Geometry: final body of the model. Coordinates: model frame, mm. A direction names the side the tool comes from. Round coordinates to 2 decimals unless told otherwise and drop trailing zeros. Write each loop counter-clockwise with the first axis right and the second up, starting at its lowest first coordinate (ties: lowest second). Pieces come first, ordered by that corner, then holes. Notation, with made-up numbers: (78.5, 38) -> (89.5, 38) arc R13 ccw to (89.5, 44) -> close; hole circle Ø7 at (2, 17.5). An arc over 180 degrees is marked (long way). Use one line per item in the form item = value. Start each with the question number.
1. Cut plane C-C, the plane x = 11. Return the cut outline in (y, z).
2. Line query: L1, parallel to Y at x = 16.5, z = 3.5; L2, parallel to X at y = 63, z = 5; L3, parallel to Y at x = -1.5, z = 4.5. Output: solid intervals per line, ascending.
3. Cut plane B-B, the plane x = 0. Return the cut outline in (y, z), plus the area to 3 significant figures.
4. Reachability of faces 1 (the face through (12.22, 64.21, -17.55)), 2 (the face through (21.209, 68, 0)), 3 (the face through (20.871, 63.634, 20.891)) from +Z, -Z, +X, -X, +Y, -Y: full face, straight path, thin tool, end or side. Return the list, or none.
5. Cut plane D-D, the plane z = 8. Return the cut outline in (x, y), plus the area to 3 significant figures.
6. Draft query along Z for faces 4 (the face through (8.598, 64, 0)), 5 (the face through (-21.209, 68, 0)), 6 (the face through (0.3, 63.6, -21.2)), 7 (the face through (0, 0, 0)). Return one class per face: pulls with the +Z half, pulls with the -Z half, needs draft (parallel to the pull), parting line crosses it, or undercut.
7. Pin query (flat end, axial travel): pin 1 Ø4 at (x, z) = (8.5, -3.5) entering from -Y; pin 2 Ø5 at (x, y) = (-2, 61.5) entering from -Z; pin 3 Ø2 at (x, z) = (-17.5, 14.5) entering from +Y. Return the tip coordinate at first contact, or that it passes through.
8. Cut plane A-A, the plane z = 0. State how many separate pieces and enclosed holes the cut face has, plus the area to 3 significant figures.
```python
from build123d import *

# Parameters (mm, degrees)
SKETCH1_R           = 1.9939
BOSS_EXTRUDE1_DEPTH = 62.8904
SKETCH2_W           = 42.418
SKETCH2_H           = 42.418
SKETCH2_R           = 1.9939
BOSS_EXTRUDE2_DEPTH = 2.6797
SKETCH2_3_W         = 45.0215
SKETCH2_3_H         = 45.0215
SKETCH2_3_W_2       = 42.418
SKETCH2_3_H_2       = 42.418
BOSS_EXTRUDE3_DEPTH = 7.62
FILLET1_R           = 2.54
SKETCH3_R           = 4.318
BOSS_EXTRUDE4_DEPTH = 9.144
FILLET2_R           = 2.54
FILLET3_R           = 1.27
CHAMFER1_SIZE       = 2.54
CHAMFER1_SIZE_2     = 1.466469684


with BuildPart() as part:
    # Sketch1 → Boss-Extrude1 (new body)
    with BuildSketch(Plane(origin=(0, 0, 0), x_dir=(1, 0, 0), z_dir=(0, 1, 0))):
        with Locations(Location((0, 0, 0), (0, 0, 270))):
            Circle(SKETCH1_R)
    extrude(amount=BOSS_EXTRUDE1_DEPTH)



with BuildPart() as body_2:
    # Sketch2 → Boss-Extrude2 (new body)
    # profile 1 of 2: a face of its own
    with BuildSketch(Plane(origin=(0, 62.8904, 0), x_dir=(1, 0, 0), z_dir=(0, 1, 0))):
        Rectangle(SKETCH2_W, SKETCH2_H)
        with Locations(Location((0, 0, 0), (0, 0, 270))):
            Circle(SKETCH2_R, mode=Mode.SUBTRACT)
        with BuildLine():
            ThreePointArc((-16.0147, -13.843), (-12.3063, -17.5514), (-8.5979, -13.843))
            Line((-8.5979, -13.843), (-8.5979, 13.843))
            ThreePointArc((-8.5979, 13.843), (-12.3063, 17.5514), (-16.0147, 13.843))
            Line((-16.0147, 13.843), (-16.0147, -13.843))
        make_face(mode=Mode.SUBTRACT)
        with BuildLine():
            Line((16.0147, 13.843), (16.0147, -13.843))
            ThreePointArc((16.0147, -13.843), (12.3063, -17.5514), (8.5979, -13.843))
            Line((8.5979, -13.843), (8.5979, 13.843))
            ThreePointArc((8.5979, 13.843), (12.3063, 17.5514), (16.0147, 13.843))
        make_face(mode=Mode.SUBTRACT)
    # profile 2 of 2: a face of its own
    with BuildSketch(Plane(origin=(0, 62.8904, 0), x_dir=(1, 0, 0), z_dir=(0, 1, 0))):
        with Locations(Location((0, 0, 0), (0, 0, 270))):
            Circle(SKETCH2_R)
    extrude(amount=BOSS_EXTRUDE2_DEPTH)


with BuildPart() as part_1:
    add(part.part)

    add(body_2.part)  # Boss-Extrude3 merges body 2
    # Sketch2<3> → Boss-Extrude3 (add)
    with BuildSketch(Plane(origin=(0, 62.8904, 0), x_dir=(1, 0, 0), z_dir=(0, 1, 0))):
        Rectangle(SKETCH2_3_W, SKETCH2_3_H)
        Rectangle(SKETCH2_3_W_2, SKETCH2_3_H_2, mode=Mode.SUBTRACT)
    extrude(amount=BOSS_EXTRUDE3_DEPTH)

    # Fillet1
    fillet1_edges = [part_1.edges().sort_by_distance(p)[0] for p in [
        (21.209, 68.04025, 21.209),
        (-21.209, 68.04025, 21.209),
        (-21.209, 68.04025, -21.209),
        (-22.51075, 66.7004, 22.51075),
        (22.51075, 66.7004, 22.51075),
        (22.51075, 66.7004, -22.51075),
        (-22.51075, 66.7004, -22.51075),
        (21.209, 68.04025, -21.209),
    ]]
    fillet(fillet1_edges, radius=FILLET1_R)

    # Sketch3 → Boss-Extrude4 (add)
    with BuildSketch(Plane.XZ.offset(-62.8904)):
        with Locations(Location((0, 0, 0), (0, 0, 90))):
            Circle(SKETCH3_R)
    extrude(amount=BOSS_EXTRUDE4_DEPTH)

    # Fillet2
    fillet2_edges = [part_1.edges().sort_by_distance(p)[0] for p in [
        (0, 62.8904, -4.318),
    ]]
    fillet(fillet2_edges, radius=FILLET2_R)

    # Fillet3
    fillet3_edges = [part_1.edges().sort_by_distance(p)[0] for p in [
        (0, 53.7464, -4.318),
    ]]
    fillet(fillet3_edges, radius=FILLET3_R)

    # Chamfer1
    # the kernel refuses this chamfer: 2.54, 1.466469684 mm, written as the material it takes off along each edge
    with BuildSketch(Plane(origin=(-19.97075, 62.8904, 22.51075), x_dir=(0, 0, -1), z_dir=(1, 0, 0)), Plane(origin=(-22.51075, 62.8904, -19.97075), x_dir=(1, 0, 0), z_dir=(0, 0, 1)), Plane(origin=(19.97075, 62.8904, -22.51075), x_dir=(0, 0, 1), z_dir=(-1, 0, 0)), Plane(origin=(22.51075, 62.8904, 19.97075), x_dir=(-1, 0, 0), z_dir=(0, 0, -1))) as chamfer1_piece_1:
        Polygon((CHAMFER1_SIZE, 0), (0, CHAMFER1_SIZE_2), (0, 0), align=None)
    extrude(amount=39.9415, mode=Mode.SUBTRACT)
    with BuildSketch(Plane(origin=(-19.97075, 62.8904, -19.97075), x_dir=(0, 0, -1), z_dir=(1, 0, 0))) as chamfer1_piece_2:
        Polygon((2.54 - CHAMFER1_SIZE, 0), (2.54, CHAMFER1_SIZE_2), (2.54, 0), align=None)
    revolve(axis=Axis((-19.97075, 62.8904, -19.97075), (0, 1, 0)), revolution_arc=90, mode=Mode.SUBTRACT)
    with BuildSketch(Plane(origin=(19.97075, 62.8904, 19.97075), x_dir=(0, 0, 1), z_dir=(-1, 0, 0))) as chamfer1_piece_3:
        Polygon((2.54 - CHAMFER1_SIZE, 0), (2.54, CHAMFER1_SIZE_2), (2.54, 0), align=None)
    revolve(axis=Axis((19.97075, 62.8904, 19.97075), (0, 1, 0)), revolution_arc=90, mode=Mode.SUBTRACT)
    with BuildSketch(Plane(origin=(19.97075, 62.8904, -19.97075), x_dir=(1, 0, 0), z_dir=(0, 0, 1))) as chamfer1_piece_4:
        Polygon((2.54 - CHAMFER1_SIZE, 0), (2.54, CHAMFER1_SIZE_2), (2.54, 0), align=None)
    revolve(axis=Axis((19.97075, 62.8904, -19.97075), (0, 1, 0)), revolution_arc=90, mode=Mode.SUBTRACT)
    with BuildSketch(Plane(origin=(-19.97075, 62.8904, 19.97075), x_dir=(0, 0, 1), z_dir=(1, 0, 0))) as chamfer1_piece_5:
        Polygon((2.54 - CHAMFER1_SIZE, 0), (2.54, -CHAMFER1_SIZE_2), (2.54, 0), align=None)
    revolve(axis=Axis((-19.97075, 62.8904, 19.97075), (0, -1, 0)), revolution_arc=90, mode=Mode.SUBTRACT)


solid = part_1.part
```
Outcome:
q1.outline = (62.89, -19.97) -> (64.36, -22.51) -> (70.51, -22.51) -> (70.51, -21.21) -> (65.57, -21.21) -> (65.57, -17.31) -> (62.89, -17.31) -> close; (62.89, 17.31) -> (65.57, 17.31) -> (65.57, 21.21) -> (70.51, 21.21) -> (70.51, 22.51) -> (64.36, 22.51) -> (62.89, 19.97) -> close
q2.L1 = 62.89 to 65.57
q2.L2 = -20.16 to -16.01, -8.6 to 8.6, 16.01 to 20.16
q2.L3 = 61.76 to 65.57
q3.outline = (0, -1.99) -> (53.75, -1.99) -> (53.75, -3.05) arc R1.27 ccw to (55.02, -4.32) -> (60.35, -4.32) arc R2.54 cw to (62.89, -6.86) -> (62.89, -19.97) -> (64.36, -22.51) -> (70.51, -22.51) -> (70.51, -21.21) -> (65.57, -21.21) -> (65.57, 21.21) -> (70.51, 21.21) -> (70.51, 22.51) -> (64.36, 22.51) -> (62.89, 19.97) -> (62.89, 6.86) arc R2.54 cw to (60.35, 4.32) -> (55.02, 4.32) arc R1.27 ccw to (53.75, 3.05) -> (53.75, 1.99) -> (0, 1.99) -> close
q3.area = 425 mm^2
q4.face_1 = +Y, -Y
q4.face_2 = +Y
q4.face_3 = +Z, +X, -Y
q5.outline = (-22.51, 64.36) -> (-19.97, 62.89) -> (-16.01, 62.89) -> (-16.01, 65.57) -> (-21.21, 65.57) -> (-21.21, 70.51) -> (-22.51, 70.51) -> close; (-8.6, 62.89) -> (8.6, 62.89) -> (8.6, 65.57) -> (-8.6, 65.57) -> close; (16.01, 62.89) -> (19.97, 62.89) -> (22.51, 64.36) -> (22.51, 70.51) -> (21.21, 70.51) -> (21.21, 65.57) -> (16.01, 65.57) -> close
q5.area = 90.0 mm^2
q6.face_4 = undercut
q6.face_5 = undercut
q6.face_6 = pulls with the -Z half
q6.face_7 = needs draft
q7.pin_1 = 62.89
q7.pin_2 = -21.89
q7.pin_3 = 65.57
q8.separate_pieces = 3
q8.enclosed_holes = 0
q8.area = 385 mm^2
